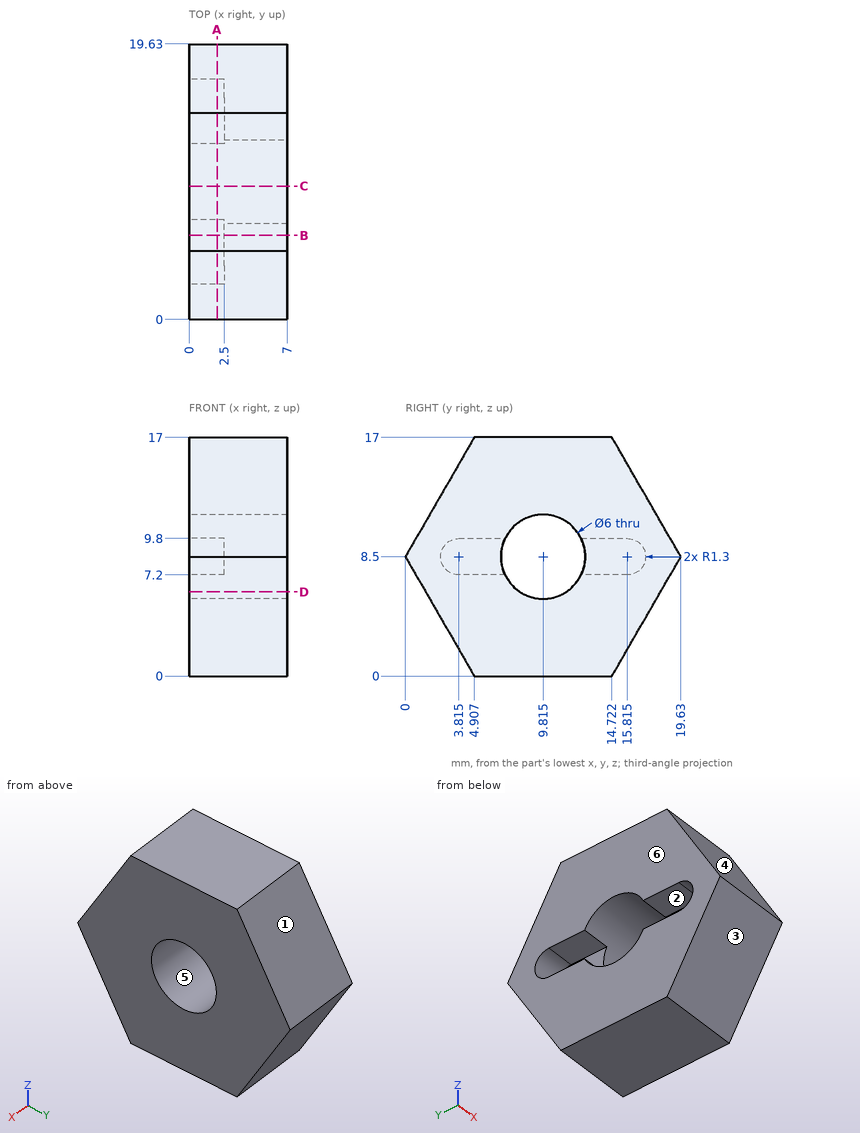
Design review of the part shown in the three views and the two pictorial views. Dimensions are in mm from the part's minimum x, y and z. A direction names the side the tool comes from. Give positions to 0.01 mm unless a question says otherwise; leave off trailing zeros. Write each loop counter-clockwise with the first axis right and the second up, starting at its lowest first coordinate (ties: lowest second). Pieces come first, ordered by that corner, then holes.
(1) Add section A-A (x = 2). Give the boundary of the cut face in (y, z) (1 decimal), and give its area (3 significant figures).
Checked values:
outline: (0, 8.5) - (4.9, 0) - (14.7, 0) - (19.6, 8.5) - (14.7, 17) - (4.9, 17) - close; hole (3.8, 7.2) - (7.1, 7.2) arc R3 ccw to (12.5, 7.2) - (15.8, 7.2) arc R1.3 ccw to (15.8, 9.8) - (12.5, 9.8) arc R3 ccw to (7.1, 9.8) - (3.8, 9.8) arc R1.3 ccw to start
area: 201 mm2
(2) Add section D-D (z = 6). Give the boundary of the cut face in (x, y).
Checked values:
outline: (0, 1.44) - (7, 1.44) - (7, 8.16) - (0, 8.16) - close; (0, 11.47) - (7, 11.47) - (7, 18.19) - (0, 18.19) - close
(3) Wall thickness on line 1 along Z through (x, y) = (1.75, 7.5) (1 decimal); line 2 along Z through (x, y) = (0.75, 8.5) (1 decimal); line 3 along Y through (x, z) = (1.25, 2.25): over which ranges is each line inside the solid? List them lowest first.
Checked values:
line 1: z = 0 to 6.6, 10.4 to 17
line 2: z = 0 to 5.8, 11.2 to 17
line 3: y = 3.61 to 16.02
(4) Tool access review of the marked faces 1 and 2: name each direction out of +Z, -Z, +X, -X, +Y, -Y from which nothing blocks a thin tool from reaching the whole face with its end or side.
Checked values:
face 1: +Z, +X, -X, +Y
face 2: -X
(5) Add section B-B (y = 6). Give the boundary of the cut face in (x, z).
Checked values:
outline: (0, 0) - (7, 0) - (7, 17) - (0, 17) - (0, 9.8) - (2.5, 9.8) - (2.5, 7.2) - (0, 7.2) - close
(6) Clearance check with a flat-ended pin moving along its axis: pin 1 Ø1 at (x, z) = (5.5, 11) entering from -Y (1 decimal). State where the tip first meets the part, or that it passes through.
Checked values:
pin 1: stops at y = 1.2
(7) Mouldability with a two-part tool opening along Z and no side actions: class the marked faces 3, 4, 5 and 6 as +Z half, -Z half, draft (parallel to the pull), parting line (faces both ways), or undercut.
Checked values:
face 3: -Z half
face 4: +Z half
face 5: undercut
face 6: draft
(8) Add section C-C (y = 9.5). Give the boundary of the cut face in (x, z).
Checked values:
outline: (0, 0) - (7, 0) - (7, 5.52) - (0, 5.52) - close; (0, 11.48) - (7, 11.48) - (7, 17) - (0, 17) - close
